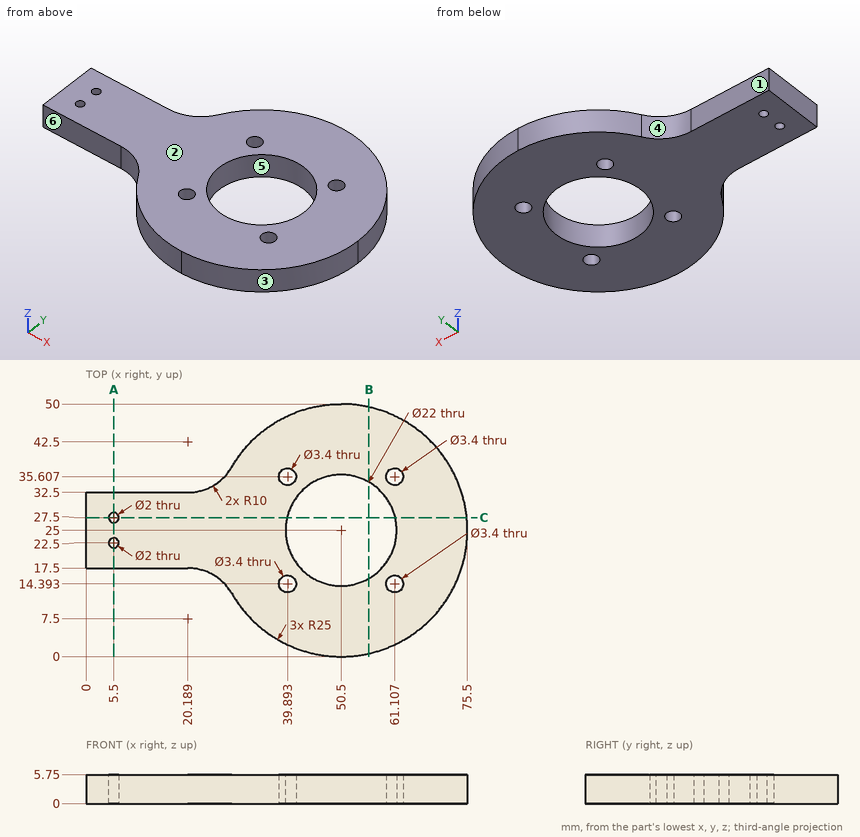
Input: dimensioned drawing with shaded views. Units: mm. Origin: part minimum x, y, z. A direction names the side the tool comes from. Round coordinates to 2 decimals unless told otherwise and drop trailing zeros. Loops run counter-clockwise (first coordinate to the right, second up) from the corner with the lowest first, then second, coordinate; pieces in that order, holes last. Notation, with made-up numbers: M 36,61 L 79,61 A30 cw 79,86 Z; hole C 48.5,-36 d11. An arc over 180 degrees is marked long. Return JSON: item names as keys, results as strings. Group by question number.
1. Section query A-A on x = 5.5. Output: boundary loops of the cut face in (y, z).
2. Section query B-B on x = 56. Output: boundary loops of the cut face in (y, z), and give its area (3 significant figures).
3. Reachability of the marked faces 1 and 2 from +Z, -Z, +X, -X, +Y, -Y: full face, straight path, thin tool, end or side. Return the list, or none.
4. Pin query (flat end, axial travel): pin 1 (1 mm diameter, centred on y = 29.5, z = 5, fed in from +X); pin 2 (1.5 mm diameter, centred on x = 49.5, z = 1, fed in from -Y); pin 3 (1.7 mm diameter, centred on x = 10.5, z = 4, fed in from +Y). Return the tip coordinate at first contact, or that it passes through.
5. Section query C-C on y = 27.5. State how many separate pieces and enclosed holes the cut face has, and give its area (3 significant figures).
6. Mould query, pull axis X, two halves, no side actions, for the marked faces 3, 4, 5 and 6. Classes: released by +X, released by -X, zero draft, split by the parting line, or undercut.
7. Material intervals for line 1 along Y through (x, z) = (5.5, 1.4); line 2 along Y through (x, z) = (39, 1.5); line 3 along Y through (x, z) = (7.5, 2.85), sorted ascending. Write a range as from..to.
Checks:
{
 "1": {"outline": "M 17.5,0 L 21.5,0 L 21.5,5.75 L 17.5,5.75 Z; M 23.5,0 L 26.5,0 L 26.5,5.75 L 23.5,5.75 Z; M 28.5,0 L 32.5,0 L 32.5,5.75 L 28.5,5.75 Z"},
 "2": {"outline": "M 0.61,0 L 15.47,0 L 15.47,5.75 L 0.61,5.75 Z; M 34.53,0 L 49.39,0 L 49.39,5.75 L 34.53,5.75 Z", "area": "171 mm²"},
 "3": {"face 1": "+Z, -Z, -X, +Y", "face 2": "+Z, +X, -X, +Y, -Y"},
 "4": {"pin 1": "stops at x = 75.18", "pin 2": "stops at y = 0", "pin 3": "stops at y = 32.5"},
 "5": {"separate pieces": "3", "enclosed holes": "0", "area": "299 mm²"},
 "6": {"face 3": "released by +X", "face 4": "released by -X", "face 5": "undercut", "face 6": "zero draft"},
 "7": {"line 1": "y = 17.5..21.5, 23.5..26.5, 28.5..32.5", "line 2": "y = 2.8..12.95, 15.84..34.16, 37.05..47.2", "line 3": "y = 17.5..32.5"}
}
